Job drawing, mm, ordinate dimensions from the low corner. One solid piece. Give positions to 0.01 mm unless a question says otherwise; leave off trailing zeros. Order: outer loops, then holes, each group sorted by start corner. A loop starts at its lowest first (then second) coordinate and runs counter-clockwise, first axis right, second up. Notation, with made-up numbers: (-4, 36) - (5, 36) arc R27 ccw to (5, 52) - close; hole circle Ø11 at (-22, 59). An arc over 180 degrees is marked (long way). Write each question's results on one line, items separated by ' | '. Start each with the question number.
1) Drop flat-ended pins along their axis: pin 1 Ø10 at (x, y) = (164.5, 28.5) entering from -Z; pin 2 Ø1.5 at (y, z) = (64.5, 8.5) entering from -X. Give the stop position or say it passes through.
2) Cut at B-B on x = 73. List the corners of the cut face in (y, z).
3) Cut at C-C on y = 63.5. List the corners of the cut face in (x, z).
4) Cut at A-A on z = 6.5. List the corners of the cut face in (x, y).
5) Drill centre lines: line 1 along Y through (x, z) = (99.5, 3.5); line 2 along X through (y, z) = (103, 0.5) (1 decimal); line 3 along X through (y, z) = (85, 10.75). Where is each one in solid material? Low to high. Write a range as from..to.
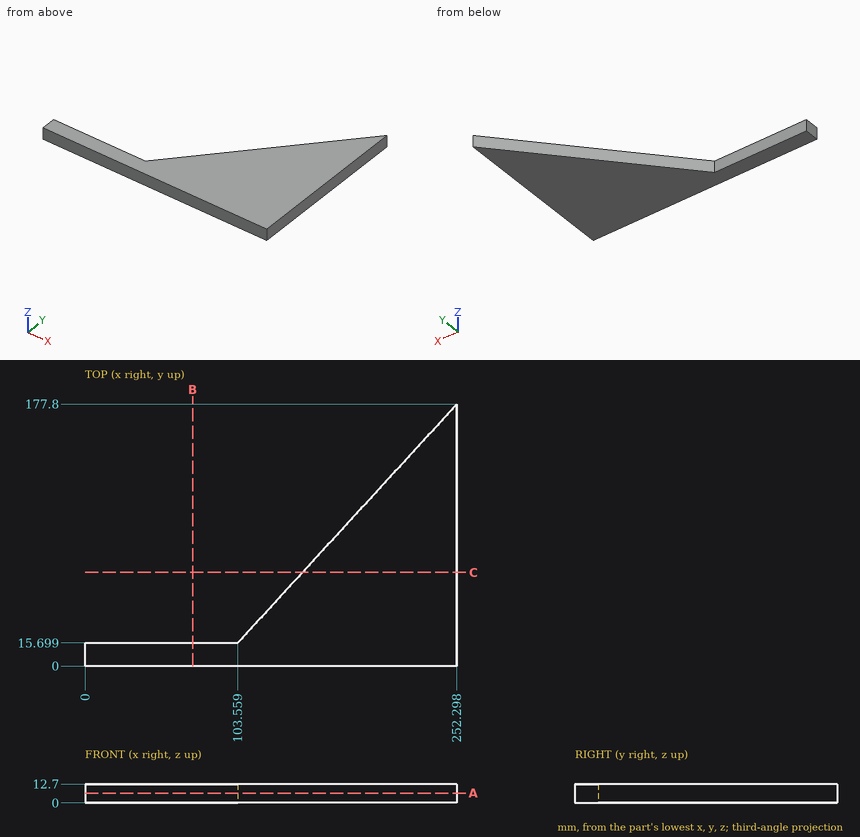
Results:
1) pin 1: z = 0 | pin 2: x = 147.65
2) outline: (0, 0) - (15.7, 0) - (15.7, 12.7) - (0, 12.7) - close
3) outline: (147.42, 0) - (252.3, 0) - (252.3, 12.7) - (147.42, 12.7) - close
4) outline: (0, 0) - (252.3, 0) - (252.3, 177.8) - (103.56, 15.7) - (0, 15.7) - close
5) line 1: 0..15.7 | line 2: 183.7..252.3 | line 3: 167.15..252.3
